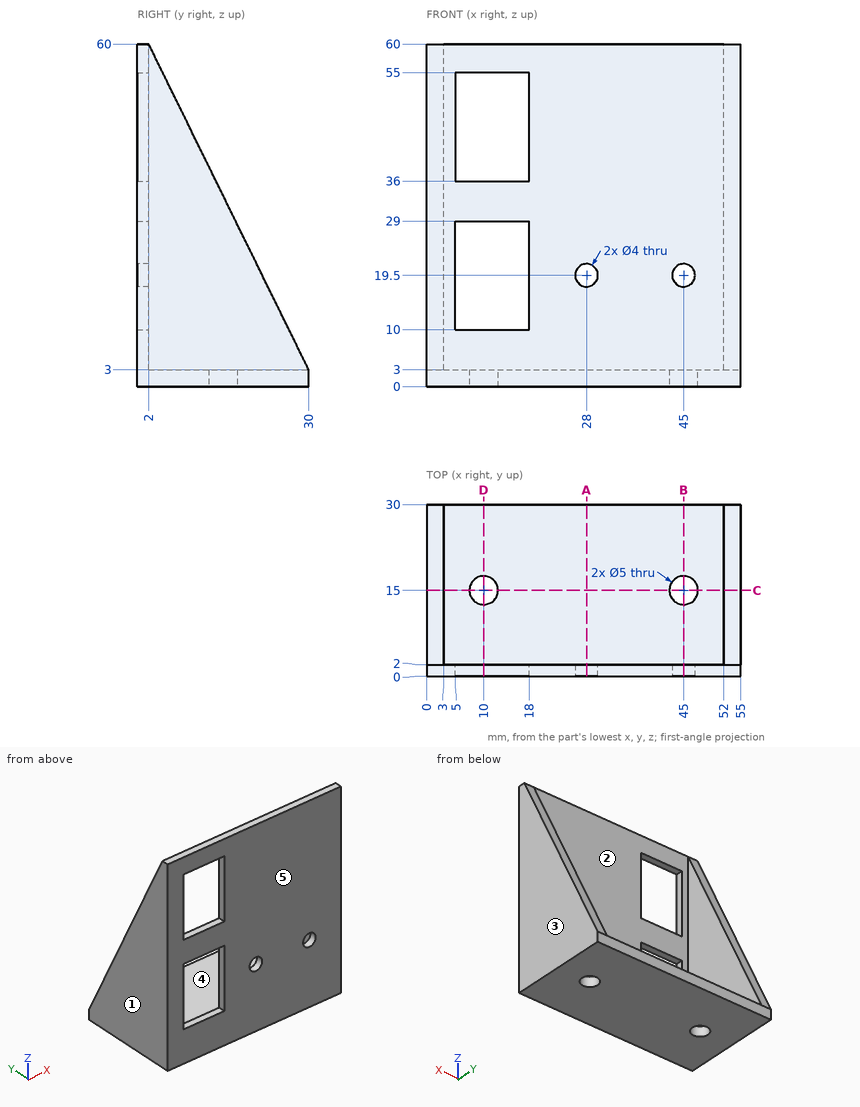
Verification items for this drawing (mm, ordinates from the low corner). A direction names the side the tool comes from. Coordinates: 2 decimals unless noted, no trailing zeros. Order: outer loops, then holes, each group sorted by start corner. A loop starts at its lowest first (then second) coordinate and runs counter-clockwise, first axis right, second up. Notation, with made-up numbers: M 65,53.5 L 94,53.5 A15 ccw 94,67.5 Z; hole C 30.5,-16 d1. An arc over 180 degrees is marked long. One line per item, written item: value. Start each with the question number.
Item 1: Access from +Z, -Z, +X, -X, +Y, -Y to the whole of each face (thin tool, end or side, straight path). Record for the marked faces 4 and 5.
Item 2: Sectioned sample at D-D on x = 10. Record the cut outline in (y, z).
Item 3: Depth check by flat-ended pin: P1, Ø8.5, axis at x = 33.5, y = 17, coming from the +Z side; P2, Ø10, axis at x = 44, z = 39.5, coming from the +Y side. Enter the tip coordinate at first touch or a pass-through.
Item 4: Sectioned sample at B-B on x = 45. Record the cut outline in (y, z).
Item 5: Sectioned sample at C-C on y = 15. Record the cut outline in (x, z).
Item 6: Thickness scan on probe 1 along Z at (x, y) = (45, 0.8); probe 2 along Y at (x, z) = (32, 32); probe 3 along Z at (x, y) = (7, 27.5). Record the ranges inside material, lowest first.
Item 7: Mould release check, pull along X, two halves, no side actions. Record for the marked faces 1, 2 and 3: pulls with the +X half, pulls with the -X half, needs draft (parallel to the pull), parting line crosses it, or undercut.
Item 8: Sectioned sample at A-A on x = 28. Record the cut outline in (y, z).
Calculated:
1. face 4: +Z, +Y
1. face 5: +Z, -Z, +X, -X, -Y
2. outline: M 0,0 L 12.5,0 L 12.5,3 L 2,3 L 2,10 L 0,10 Z; M 0,29 L 2,29 L 2,36 L 0,36 Z; M 0,55 L 2,55 L 2,60 L 0,60 Z; M 17.5,0 L 30,0 L 30,3 L 17.5,3 Z
3. P1: z = 3
3. P2: y = 2
4. outline: M 0,0 L 12.5,0 L 12.5,3 L 2,3 L 2,17.5 L 0,17.5 Z; M 0,21.5 L 2,21.5 L 2,60 L 0,60 Z; M 17.5,0 L 30,0 L 30,3 L 17.5,3 Z
5. outline: M 0,0 L 7.5,0 L 7.5,3 L 3,3 L 3,33.54 L 0,33.54 Z; M 12.5,0 L 42.5,0 L 42.5,3 L 12.5,3 Z; M 47.5,0 L 55,0 L 55,33.54 L 52,33.54 L 52,3 L 47.5,3 Z
6. probe 1: 0 to 17.5, 21.5 to 60
6. probe 2: 0 to 2
6. probe 3: 0 to 3
7. face 1: pulls with the -X half
7. face 2: undercut
7. face 3: pulls with the +X half
8. outline: M 0,0 L 30,0 L 30,3 L 2,3 L 2,17.5 L 0,17.5 Z; M 0,21.5 L 2,21.5 L 2,60 L 0,60 Z
